```python
from build123d import *

# Parameters (mm, degrees)
SKETCH2_W           = 77
SKETCH2_H           = 45
SKETCH2_R           = 2.1
BOSS_EXTRUDE2_DEPTH = 20
CUT_EXTRUDE1_DEPTH  = 15
SKETCH4_R           = 2.1
SKETCH4_W           = 52.379694286
SKETCH4_H           = 20.484576037
SKETCH4_W_2         = 36.58107182
SKETCH4_H_2         = 18.515423963
SKETCH4_W_3         = 13.798622466
SKETCH4_H_3         = 16.515423963
SKETCH4_W_4         = 8.316970937
SKETCH4_H_4         = 22.484576037
SKETCH4_W_5         = 8.303334777
SKETCH4_H_5         = 20.515423963
CUT_EXTRUDE2_DEPTH  = 3
CUT_EXTRUDE3_REACH  = 79
FILLET1_R           = 2
CUT_EXTRUDE8_DEPTH  = 20
CHAMFER1_SIZE       = 0.3


with BuildPart() as part:
    # Sketch2 → Boss-Extrude2 (new body)
    with BuildSketch(Plane.XY):
        with Locations((30.99874, -9.99994)):
            Rectangle(SKETCH2_W, SKETCH2_H)
        with Locations((-0.00126, 6e-05)):
            Circle(SKETCH2_R, mode=Mode.SUBTRACT)
        with Locations((61.99874, -19.99994)):
            Circle(SKETCH2_R, mode=Mode.SUBTRACT)
    extrude(amount=BOSS_EXTRUDE2_DEPTH)

    # Sketch3 → Cut-Extrude1 (cut)
    with BuildSketch(Plane.XY.offset(20)):
        Polygon((-5.50126, 10.50006), (67.49874, 10.50006), (67.49874, -30.49994), (-0.50126, -30.49994), (-0.50126, -10.49994), (-5.50126, -10.49994), align=None)
    extrude(amount=-CUT_EXTRUDE1_DEPTH, mode=Mode.SUBTRACT)

    # Sketch4 → Cut-Extrude2 (cut)
    with BuildSketch(Plane.XY.offset(5)):
        with Locations((-0.00126, 6e-05)):
            Circle(SKETCH4_R)
        with Locations((61.99874, -19.99994)):
            Circle(SKETCH4_R)
        with Locations((30.99192192, 0.257771982)):
            Rectangle(SKETCH4_W, SKETCH4_H)
        with Locations((23.092610687, -21.242228019)):
            Rectangle(SKETCH4_W_2, SKETCH4_H_2)
        with Locations((50.28245783, -20.242228019)):
            Rectangle(SKETCH4_W_3, SKETCH4_H_3)
        with Locations((63.340254532, -0.742228018)):
            Rectangle(SKETCH4_W_4, SKETCH4_H_4)
        with Locations((-1.349592612, -20.242228019)):
            Rectangle(SKETCH4_W_5, SKETCH4_H_5)
    extrude(amount=-CUT_EXTRUDE2_DEPTH, mode=Mode.SUBTRACT)

    # Sketch5 → Cut-Extrude3 (cut, up to next)
    with BuildSketch(Plane.ZY.offset(7.50126), mode=Mode.PRIVATE) as cut_extrude3_sk1:
        with BuildLine():
            Line((10, -12.49994), (15, -12.49994))
            ThreePointArc((15, -12.49994), (16.414213562, -13.085726438), (17, -14.49994))
            Line((17, -14.49994), (17, -26.49994))
            ThreePointArc((17, -26.49994), (16.414213562, -27.914153562), (15, -28.49994))
            Line((15, -28.49994), (10, -28.49994))
            ThreePointArc((10, -28.49994), (8.585786438, -27.914153562), (8, -26.49994))
            Line((8, -26.49994), (8, -14.49994))
            ThreePointArc((8, -14.49994), (8.585786438, -13.085726438), (10, -12.49994))
        make_face()
    cut_extrude3_tool1 = extrude(cut_extrude3_sk1.sketch, amount=-CUT_EXTRUDE3_REACH, mode=Mode.PRIVATE) & part.part
    add(cut_extrude3_tool1.solids().sort_by_distance((-7.50126, -20.49994, 12.5))[0], mode=Mode.SUBTRACT)

    # Fillet1
    fillet1_edges = [part.edges().sort_by_distance(p)[0] for p in [
        (-7.50126, 12.50006, 10),
        (69.49874, 12.50006, 10),
        (69.49874, -32.49994, 10),
        (-7.50126, -32.49994, 10),
    ]]
    fillet(fillet1_edges, radius=FILLET1_R)

    # Sketch6 → Cut-Extrude8 (cut)
    with BuildSketch(Plane(origin=(0, -10.49994, 0), x_dir=(1, 0, 0), z_dir=(0, 1, 0))):
        Polygon((-5.50126, -7), (-0.50126, -11.195498156), (-0.50126, -5), (-5.50126, -5), align=None)
    extrude(amount=-CUT_EXTRUDE8_DEPTH, mode=Mode.SUBTRACT)

    # Chamfer1
    chamfer1_edges = [part.edges().sort_by_distance(p)[0] for p in [
        (-2.10126, 6e-05, 0),
        (69.49874, -9.99994, 0),
        (-7.50126, -9.99994, 0),
        (30.99874, 12.50006, 0),
        (30.99874, -32.49994, 0),
        (-6.915473562, -31.914153562, 0),
        (-6.915473562, 11.914273562, 0),
        (68.912953562, 11.914273562, 0),
        (68.912953562, -31.914153562, 0),
        (59.89874, -19.99994, 0),
    ]]
    chamfer(chamfer1_edges, length=CHAMFER1_SIZE)


solid = part.part
```
Work out the finished part from the listing and answer in its coordinate system (mm). A direction names the side the tool comes from. Round coordinates to 2 decimals unless told otherwise and drop trailing zeros. Write each loop counter-clockwise with the first axis right and the second up, starting at its lowest first coordinate (ties: lowest second). Pieces come first, ordered by that corner, then holes.
1) Flat-ended cylindrical pins translate along their axes: P1, Ø4, axis at x = 2.5, y = -24, coming from the +Z side; P2, Ø7, axis at x = 49.5, y = -18, coming from the +Z side. Find the tip coordinate at first contact, or state that the pin passes through.
2) Determine the mould class of faces 5 (the face through (68.897, -31.93, 10.288)), 6 (the face through (-4.05, -27.9, 16.43)), 7 (the face through (31, 0, 2)) for opening direction Z: pulls with the +Z half, pulls with the -Z half, needs draft (parallel to the pull), parting line crosses it, or undercut.
3) A cutting plane is placed at C-C on x = 35. Determine the outline of the cut face in (y, z).
4) A cutting plane is placed at D-D on y = 6. Determine the outline of the cut face in (x, z).
5) Consider probe 1 along X at (y, z) = (-4, 4); probe 2 along X at (y, z) = (-12.5, 3.25); probe 3 along Y at (x, z) = (7, 10). Determine where each line is inside the solid, lowest interval first.
6) A cutting plane is placed at A-A on y = -23.5. Determine the outline of the cut face in (x, z).
7) A cutting plane is placed at B-B on z = 12. Determine the outline of the cut face in (x, y).
8) Which of the six approach directions +Z, -Z, +X, -X, +Y, -Y give full straight-line access (tool end or side, diameter ignored) to faces 1 (the face through (4.802, 0, 4)), 2 (the face through (68.897, 11.93, 10.288)), 3 (the face through (-5.501, -6, 11)), 4 (the face through (-4, -28.5, 13))?
Entries:
1. P1: stops at z = 5
1. P2: stops at z = 2
2. face 5: needs draft
2. face 6: undercut
2. face 7: pulls with the +Z half
3. outline: (-32.5, 0.3) - (-32.2, 0) - (12.2, 0) - (12.5, 0.3) - (12.5, 20) - (10.5, 20) - (10.5, 2) - (-9.98, 2) - (-9.98, 5) - (-11.98, 5) - (-11.98, 2) - (-30.5, 2) - (-30.5, 20) - (-32.5, 20) - close
4. outline: (-7.5, 0.3) - (-7.2, 0) - (69.2, 0) - (69.5, 0.3) - (69.5, 20) - (67.5, 20) - (67.5, 2) - (59.18, 2) - (59.18, 5) - (57.18, 5) - (57.18, 2) - (4.8, 2) - (4.8, 5) - (-5.5, 5) - (-5.5, 20) - (-7.5, 20) - close
5. probe 1: x = -7.5 to 4.8, 57.18 to 59.18, 67.5 to 69.5
5. probe 2: x = -7.5 to -5.5, 2.8 to 4.8, 41.38 to 43.38, 57.18 to 69.5
5. probe 3: y = -32.5 to -30.5, 10.5 to 12.5
6. outline: (-7.5, 0.3) - (-7.2, 0) - (69.2, 0) - (69.5, 0.3) - (69.5, 20) - (67.5, 20) - (67.5, 5) - (57.18, 5) - (57.18, 2) - (43.38, 2) - (43.38, 5) - (41.38, 5) - (41.38, 2) - (4.8, 2) - (4.8, 5) - (2.8, 5) - (2.8, 2) - (-5.5, 2) - (-5.5, 7) - (-4.31, 8) - (-7.5, 8) - close; (-7.5, 17) - (-0.5, 17) - (-0.5, 20) - (-7.5, 20) - close
7. outline: (-7.5, -30.5) arc R2 ccw to (-5.5, -32.5) - (67.5, -32.5) arc R2 ccw to (69.5, -30.5) - (69.5, 10.5) arc R2 ccw to (67.5, 12.5) - (-5.5, 12.5) arc R2 ccw to (-7.5, 10.5) - (-7.5, -12.5) - (-0.5, -12.5) - (-0.5, -10.5) - (-5.5, -10.5) - (-5.5, 10.5) - (67.5, 10.5) - (67.5, -30.5) - (-0.5, -30.5) - (-0.5, -28.5) - (-7.5, -28.5) - close
8. face 1: +Z
8. face 2: +Z, -Z, +X, +Y
8. face 3: none
8. face 4: -X
